Geometry check sheet. Reference: drawing and pictorial views, mm from the part's lowest x, y, z. Round coordinates to 2 decimals unless told otherwise and drop trailing zeros. Loops run counter-clockwise (first coordinate to the right, second up) from the corner with the lowest first, then second, coordinate; pieces in that order, holes last. Notation, with made-up numbers: (48, 39) -> (62, 39) arc R18 cw to (62, 62) -> close; hole circle Ø4 at (-11.75, 72). An arc over 180 degrees is marked (long way). Use one line per item in the form item = value.
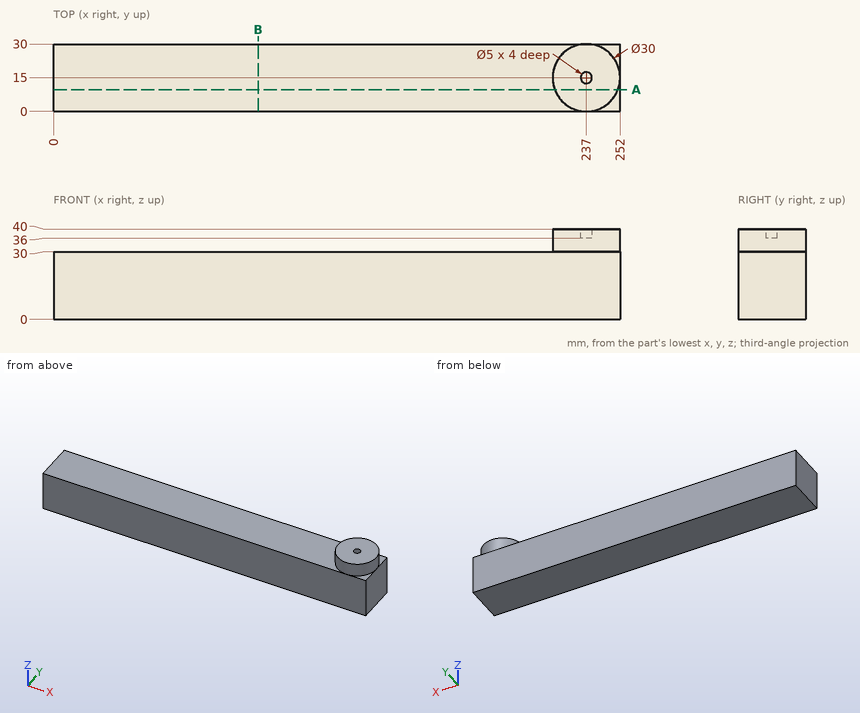
1. Section check B-B (x = 91). Record the boundary of the cut face in (y, z), then the cut area to 3 significant figures.
Return value:
outline = (0, 0) -> (30, 0) -> (30, 30) -> (0, 30) -> close
area = 900 mm2
2. Section check A-A (y = 9.75). Record the boundary of the cut face in (x, z).
Return value:
outline = (0, 0) -> (252, 0) -> (252, 30) -> (251.05, 30) -> (251.05, 40) -> (222.95, 40) -> (222.95, 30) -> (0, 30) -> close
3. Material ranges on line 1 along Y through (x, z) = (237, 38.55); line 2 along Z through (x, y) = (192.5, 13.25); line 3 along X through (y, z) = (26.5, 31.5), recorded low to high.
Return value:
line_1 = 0 to 12.5, 17.5 to 30
line_2 = 0 to 30
line_3 = 227.37 to 246.63
4. Gauge pin test, flat ends, axial feed: pin 1 (4.5 mm diameter, centred on x = 237, y = 15, fed in from +Z); pin 2 (15 mm diameter, centred on x = 158.5, y = 15.5, fed in from +Z). Record the tip position at first contact, or that the pin passes through.
Return value:
pin_1 = 36
pin_2 = 30
